Part print with two shaded views. Sizes in mm from the minimum x, y, z corner. Coordinates: 2 decimals unless noted, no trailing zeros. Loops run counter-clockwise (first coordinate to the right, second up) from the corner with the lowest first, then second, coordinate; pieces in that order, holes last. Notation, with made-up numbers: (77, -36.75) -> (112, -36.75) arc R22 ccw to (112, -0.75) -> close; hole circle Ø4 at (31.5, 12). An arc over 180 degrees is marked (long way). Use one line per item in the form item = value.
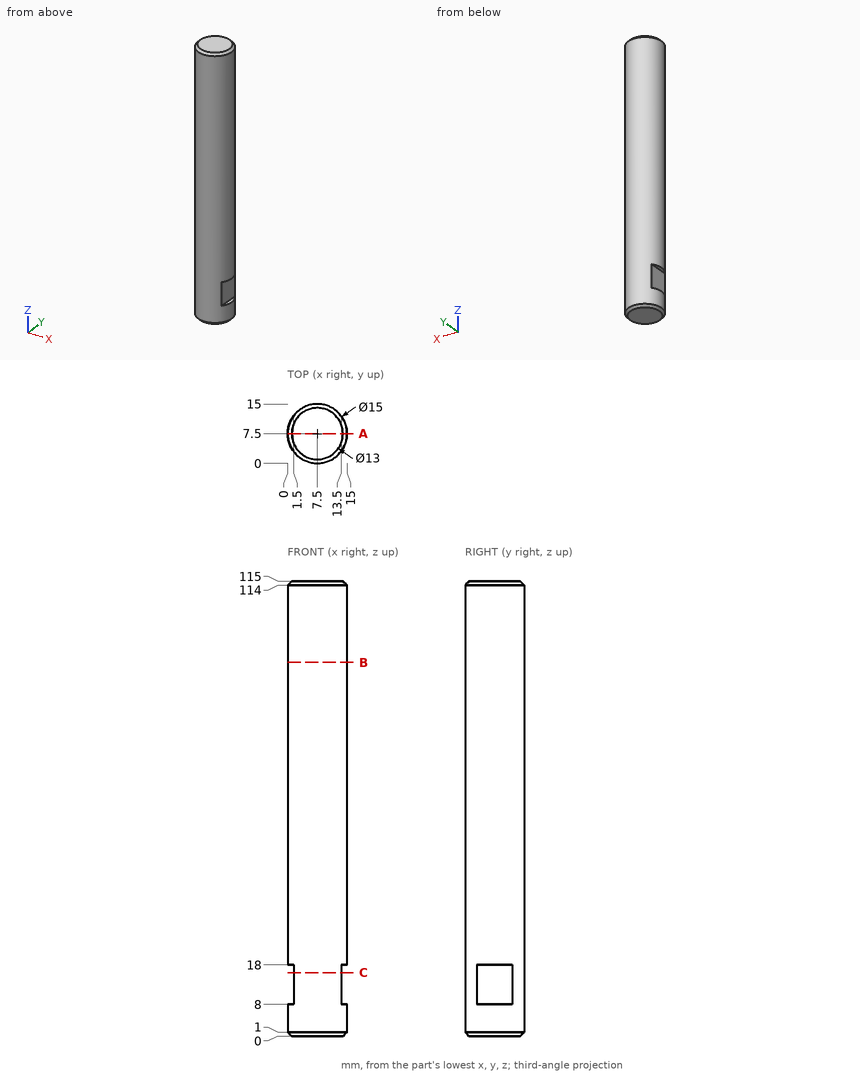
Q1. Wall check: line 1 along Y through (x, z) = (7.25, 87); line 2 along Y through (x, z) = (12, 13.5); line 3 along X through (y, z) = (1.5, 22). Give the ranges that are in metal, low to high.
Result:
line_1 = 0 to 15
line_2 = 1.5 to 13.5
line_3 = 3 to 12
Q2. Band-saw the part on A-A, the plane y = 7.5. Write the cut outline in (x, z).
Result:
outline = (0, 1) -> (1, 0) -> (14, 0) -> (15, 1) -> (15, 8) -> (13.5, 8) -> (13.5, 18) -> (15, 18) -> (15, 114) -> (14, 115) -> (1, 115) -> (0, 114) -> (0, 18) -> (1.5, 18) -> (1.5, 8) -> (0, 8) -> close
Q3. Band-saw the part on B-B, the plane z = 94.5. Write the cut outline in (x, y).
Result:
outline = circle Ø15 at (7.5, 7.5)
Q4. Band-saw the part on C-C, the plane z = 16. Write the cut outline in (x, y), and give its area (3 significant figures).
Result:
outline = (1.5, 3) arc R7.5 ccw to (13.5, 3) -> (13.5, 12) arc R7.5 ccw to (1.5, 12) -> close
area = 158 mm2
Q5. Pin check, flat tips, straight feed: pin 1 Ø1.2 at (x, y) = (14, 7.5) entering from -Z; pin 2 Ø4.5 at (y, z) = (7.5, 13) entering from +X; pin 3 Ø2.5 at (y, z) = (5.5, 14) entering from -X; pin 4 Ø6 at (y, z) = (3, 44) entering from +X. Stop position of each tip, or through.
Result:
pin_1 = 0
pin_2 = 13.5
pin_3 = 1.5
pin_4 = 14.85
